Part model, mm, in its own coordinate system. A direction names the side the tool comes from. Give positions to 0.01 mm unless a question says otherwise; leave off trailing zeros. Write each loop counter-clockwise with the first axis right and the second up, starting at its lowest first coordinate (ties: lowest second). Pieces come first, ordered by that corner, then holes. Notation, with made-up numbers: (29.25, 55) - (63.25, 55) arc R17 ccw to (63.25, 69) - close; hole circle Ø6 at (-20.75, -38.5). An arc over 180 degrees is marked (long way). Answer as a JSON object with one key per item and string values. Group by question number.
```python
from build123d import *

# Parameters (mm, degrees)
SKETCH_1_W                   = 420
SKETCH_1_H                   = 50
EXTRUDE_1_DEPTH              = 12
CHAMFER_1_SIZE               = 10
SKETCH_2_R                   = 11
CUT_EXTRUDE_1_DEPTH          = 424.135911972
SKETCH_3_R                   = 15
CUT_EXTRUDE_2_DEPTH          = 7
HOLE_WIZARD_M5_1_D           = 5.8
HOLE_WIZARD_M5_1_CBORE_D     = 10
HOLE_WIZARD_M5_1_CBORE_DEPTH = 5
HOLE_WIZARD_M5_2_D           = 5.8
HOLE_WIZARD_M5_2_CBORE_D     = 10
HOLE_WIZARD_M5_2_CBORE_DEPTH = 5
HOLE_WIZARD_M4_1_D           = 3.3
HOLE_WIZARD_M4_1_DEPTH       = 10.1
HOLE_WIZARD_M4_1_TIP         = 0.991420021


with BuildPart() as part:
    # 草图1 → 凸台-拉伸1 (new body)
    with BuildSketch(Plane.XY):
        with Locations((210, 25)):
            Rectangle(SKETCH_1_W, SKETCH_1_H)
    extrude(amount=EXTRUDE_1_DEPTH)

    # 倒角1
    chamfer_1_edges = [part.edges().sort_by_distance(p)[0] for p in [
        (0, 50, 6),
        (420, 50, 6),
    ]]
    chamfer(chamfer_1_edges, length=CHAMFER_1_SIZE)

    # 草图2 → 切除-拉伸1 (cut, through all)
    with BuildSketch(Plane.XY.offset(12)):
        with Locations((210, 30)):
            Circle(SKETCH_2_R)
    extrude(amount=-CUT_EXTRUDE_1_DEPTH, mode=Mode.SUBTRACT)

    # 草图3 → 切除-拉伸2 (cut)
    with BuildSketch(Plane(origin=(0, 0, 0), x_dir=(-1, 0, 0), z_dir=(0, 0, -1))):
        with Locations((-210, 30)):
            Circle(SKETCH_3_R)
    extrude(amount=-CUT_EXTRUDE_2_DEPTH, mode=Mode.SUBTRACT)

    # M5 六角凹头螺钉的柱形沉头孔1 (through all)
    with Locations(Plane(origin=(0, 50, 0), x_dir=(-1, 0, 0), z_dir=(0, 1, 0))):
        with Locations((-20, 6), (-160, 6), (-260, 5.528486678), (-400, 6)):
            CounterBoreHole(HOLE_WIZARD_M5_1_D / 2, HOLE_WIZARD_M5_1_CBORE_D / 2, HOLE_WIZARD_M5_1_CBORE_DEPTH)

    # M5 六角凹头螺钉的柱形沉头孔2 (through all)
    with Locations(Plane(origin=(0, 0, 0), x_dir=(-1, 0, 0), z_dir=(0, 0, -1))):
        with Locations((-287.5, 41), (-287.5, 15), (-132.5, 41), (-132.5, 15)):
            CounterBoreHole(HOLE_WIZARD_M5_2_D / 2, HOLE_WIZARD_M5_2_CBORE_D / 2, HOLE_WIZARD_M5_2_CBORE_DEPTH)

    # M4 螺纹孔1
    with Locations(Plane(origin=(0, 0, 0), x_dir=(-1, 0, 0), z_dir=(0, 0, -1))):
        with Locations((-243, 25.5), (-243, 10.5)):
            Hole(HOLE_WIZARD_M4_1_D / 2, depth=HOLE_WIZARD_M4_1_DEPTH)
            with Locations((0, 0, -(HOLE_WIZARD_M4_1_DEPTH + HOLE_WIZARD_M4_1_TIP / 2))):  # 118° drill point
                Cone(0, HOLE_WIZARD_M4_1_D / 2, HOLE_WIZARD_M4_1_TIP, mode=Mode.SUBTRACT)


solid = part.part
```
1) Drill centre lines: line 1 along Y through (x, z) = (132.5, 1.95); line 2 along Y through (x, z) = (210, 4.25); line 3 along Z through (x, y) = (260, 35). Where is each one in solid material? Low to high. Write a range as from..to.
2) Saw through at A-A (x = 215). List the corners of the cut face in (y, z), and give its area (3 significant figures).
3) Two-plate mould, pull along Y, no slides. Class faces 4 (the flat face through (397.8, 45, 3.8)), 5 (the cylindrical face through (25, 48, 6)), 6 (the flat face through (285, 39, 5)): +Y half, -Y half, draft (parallel to the pull), parting line (faces both ways), or undercut.
4) Drop flat-ended pins along their axis: P1, Ø5, axis at x = 260, z = 5.53, coming from the -Y side; P2, Ø6.5, axis at x = 287.5, y = 41, coming from the -Z side. Give the stop position or say it passes through.
5) Which spindle directions (+Z, -Z, +X, -X, +Y, -Y) get a long thin tool onto all of the face, cutting with end or side? Do faces 1 (the flat face through (5, 45, 6)), 2 (the flat face through (258, 45, 3)), 3 (the cylindrical face through (195.693, 34.506, 3.451)). Say none if no direction does.
Checks:
{
 "1": {"line 1": "0..10, 20..36, 46..50", "line 2": "0..15, 45..50", "line 3": "0..2.63, 8.43..12"},
 "2": {"outline": "(0, 0) - (15.86, 0) - (15.86, 7) - (20.2, 7) - (20.2, 12) - (0, 12) - close; (39.8, 7) - (44.14, 7) - (44.14, 0) - (50, 0) - (50, 12) - (39.8, 12) - close", "area": "304 mm2"},
 "3": {"face 4": "+Y half", "face 5": "draft", "face 6": "undercut"},
 "4": {"P1": "through", "P2": "z = 5"},
 "5": {"face 1": "+Z, -Z, -X, +Y", "face 2": "+Y", "face 3": "-Z"}
}
